from build123d import *

# Parameters (mm, degrees)
CUT_EXTRUDE_1_DEPTH      = 18.521415468
CUT_EXTRUDE_1_DEPTH_BACK = 18.521415468
SKETCH_2_R               = 0.5
FILLET_1_R               = 0.6
CHAMFER_1_SIZE           = 1
CHAMFER_1_SIZE2          = 0.577350269


with BuildPart() as part:
    # 草图1 → Revolve 549 (revolve)
    with BuildSketch(Plane.XY, mode=Mode.PRIVATE) as revolve_549_sk:
        Polygon((0, 0), (17, 0), (17, 2), (1, 2), (1, 3), (0.5, 3), (0, 2.5), align=None)
    revolve(revolve_549_sk.sketch.rotate(Axis((0, 0, 0), (-1, 0, 0)), 90), axis=Axis((0, 0, 0), (-1, 0, 0)))

    # 草图2 → 切除-拉伸1 (cut, two sides: drawn at the far end of the back side and taken through both)
    with BuildSketch(Plane.XY.offset(-CUT_EXTRUDE_1_DEPTH_BACK)):
        with Locations((14.8, 0)):
            Circle(SKETCH_2_R)
    extrude(amount=CUT_EXTRUDE_1_DEPTH + CUT_EXTRUDE_1_DEPTH_BACK, mode=Mode.SUBTRACT)

    # 圆角1
    fillet_1_edges = [part.edges().sort_by_distance(p)[0] for p in [
        (1, 0, 2),
    ]]
    fillet(fillet_1_edges, radius=FILLET_1_R)

    # 倒角1
    chamfer_1_edges = [part.edges().sort_by_distance(p)[0] for p in [
        (17, 0, 2),
    ]]
    chamfer_1_side = [part.faces().sort_by_distance(p)[0] for p in [
        (9.3, 0, 2),
    ]]
    chamfer(chamfer_1_edges, length=CHAMFER_1_SIZE, length2=CHAMFER_1_SIZE2, reference=chamfer_1_side[0])


solid = part.part
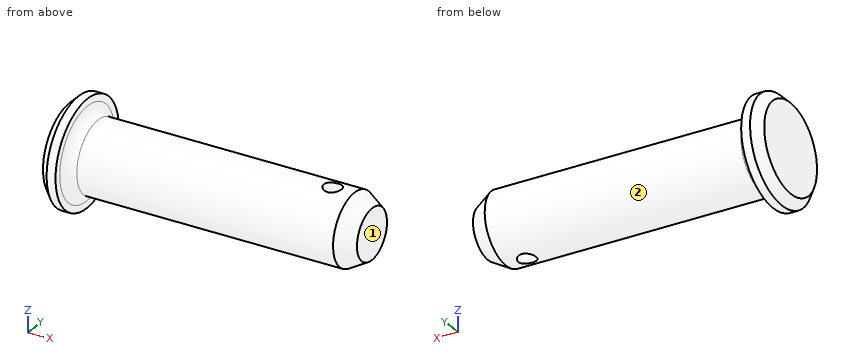
Part model, mm, in its own coordinate system. Face numbers are marked on the shaded views. A direction names the side the tool comes from. Give positions to 0.01 mm unless a question says otherwise; leave off trailing zeros. Loops run counter-clockwise (first coordinate to the right, second up) from the corner with the lowest first, then second, coordinate; pieces in that order, holes last. Notation, with made-up numbers: (32.5, -23.5) -> (57.5, -23.5) arc R19 ccw to (57.5, 7.5) -> close; hole circle Ø7 at (-13, -22.75). An arc over 180 degrees is marked (long way). Write each question's results on one line, items separated by ' | '. Start each with the question number.
Q1. Band-saw the part on C-C on x = 14.8. List the corners of the cut face in (y, z), plus the area to 3 significant figures.
Q2. Which spindle directions (+Z, -Z, +X, -X, +Y, -Y) get a long thin tool onto all of the face, cutting with end or side? Do the marked faces 1 and 2. Say none if no direction does.
Q3. Wall check: L1, parallel to X at y = 0, z = 0.5; L2, parallel to Y at x = 14.8, z = 0.05; L3, parallel to Z at x = 13, y = 0.1. Give the ranges that are in metal, low to high.
Q4. Band-saw the part on B-B on y = 0. List the corners of the cut face in (x, z), plus the area to 3 significant figures.
Q5. Band-saw the part on D-D on x = 6.75. List the corners of the cut face in (y, z), plus the area to 3 significant figures.
Q6. Band-saw the part on A-A on z = 0. List the corners of the cut face in (x, y), plus the area to 3 significant figures.
Q7. Pin check, flat tips, straight feed: P1, Ø3, axis at x = 5, y = 0.5, coming from the -Z side; P2, Ø1, axis at x = 9, z = -1.5, coming from the +Y side; P3, Ø1, axis at x = 4, z = 0, coming from the -Y side. Stop position of each tip, or through.
Results are:
1) outline: (-0.5, -1.94) -> (-0.5, 1.94) arc R2 ccw to start; (0.5, -1.94) arc R2 ccw to (0.5, 1.94) -> close | area: 8.61 mm²
2) face 1: +Z, -Z, +X, +Y, -Y | face 2: +X
3) L1: x = 0 to 14.3, 15.3 to 17 | L2: y = -2 to -0.5, 0.5 to 2 | L3: z = -2 to 2
4) outline: (0, -2.5) -> (0.5, -3) -> (1, -3) -> (1, -2.6) arc R0.6 cw to (1.6, -2) -> (14.3, -2) -> (14.3, 2) -> (1.6, 2) arc R0.6 cw to (1, 2.6) -> (1, 3) -> (0.5, 3) -> (0, 2.5) -> close; (15.3, -2) -> (16, -2) -> (17, -1.42) -> (17, 1.42) -> (16, 2) -> (15.3, 2) -> close | area: 65.3 mm²
5) outline: circle Ø4 at (0, 0) | area: 12.6 mm²
6) outline: (0, -2.5) -> (0.5, -3) -> (1, -3) -> (1, -2.6) arc R0.6 cw to (1.6, -2) -> (16, -2) -> (17, -1.42) -> (17, 1.42) -> (16, 2) -> (1.6, 2) arc R0.6 cw to (1, 2.6) -> (1, 3) -> (0.5, 3) -> (0, 2.5) -> close; hole circle Ø1 at (14.8, 0) | area: 68.5 mm²
7) P1: stops at z = -2 | P2: stops at y = 1.73 | P3: stops at y = -2
